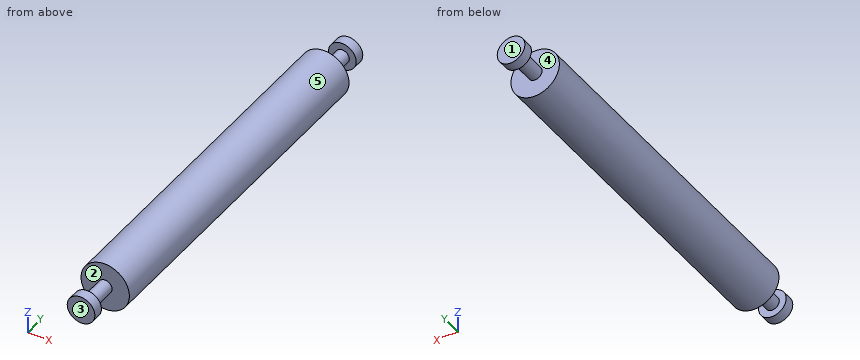
```python
from build123d import *

# Parameters (mm, degrees)
F0_R     = 3.5
F0_R_2   = 2
F0_R_3   = 1
F1_DEPTH = 25
F2_R     = 1
F3_DEPTH = 4
F4_W     = 1.5
F4_H     = 2


with BuildPart() as f1:
    # F0 (on Front) → F1 (new body)
    with BuildSketch(Plane.XZ):
        Circle(F0_R)
        Circle(F0_R_2, mode=Mode.SUBTRACT)
        Circle(F0_R_2)
        Circle(F0_R_3, mode=Mode.SUBTRACT)
        Circle(F0_R_3)
    extrude(amount=-F1_DEPTH)

    # F2 (on Front) → F3 (join)
    with BuildSketch(Plane.XZ):
        Circle(F2_R)
    extrude(amount=F3_DEPTH)

    # F4 (on Right) → F5 (revolve)
    with BuildSketch(Plane.YZ):
        with Locations((-4.75, 1)):
            Rectangle(F4_W, F4_H)
    revolve(axis=Axis((0, -4.75, 0), (0, 1, 0)))

    # F6: F1 across face


with BuildPart() as f1_1:
    add(f1.part)
    add(f1.part.mirror(Plane(origin=(0, 25, 0), x_dir=(1, 0, 0), z_dir=(0, 1, 0))))


solid = f1_1.part
```
Geometry: final body of the model. Coordinates: model frame, mm. Face numbers are marked on the shaded views. A direction names the side the tool comes from. Give positions to 0.01 mm unless a question says otherwise; leave off trailing zeros. Loops run counter-clockwise (first coordinate to the right, second up) from the corner with the lowest first, then second, coordinate; pieces in that order, holes last. Notation, with made-up numbers: (48, 84) - (91, 84) arc R14 ccw to (91, 101) - close; hole circle Ø4 at (59, -14.75). An arc over 180 degrees is marked (long way). Answer as CSV lines item,"result". Start each with the question number.
(1) Reachability of the marked faces 4 and 5 from +Z, -Z, +X, -X, +Y, -Y: full face, straight path, thin tool, end or side. Return the list, or none.
(2) Section query C-C (y = 35.5). Output: boundary loops of the cut face in (x, z).
(3) Pin query (flat end, axial travel): P1, Ø2, axis at y = 32.5, z = -2, coming from the -X side; P2, Ø1, axis at x = -2, z = -2.5, coming from the +Y side; P3, Ø2, axis at y = 11.5, z = 1.5, coming from the +X side. Return the tip coordinate at first contact, or that it passes through.
(4) Mould query, pull axis Y, two halves, no side actions, for the marked faces 1, 2 and 3. Classes: +Y half, -Y half, draft (parallel to the pull), parting line (faces both ways), or undercut.
(5) Section query A-A (x = 0). Output: boundary loops of the cut face in (y, z), and give its area (3 significant figures).
(6) Ray query, line 1 along Y through (x, z) = (-1.25, -0.75); line 2 along Y through (x, z) = (-2.5, -0.5); line 3 along Z through (x, y) = (0.25, 43). Return the intervals inside material, ascending. Write a range as [from, to].
(7) Section query B-B (z = -1.5). Output: boundary loops of the cut face in (x, y), and give its area (3 significant figures).
Worked answers:
1,face 4,"none"
1,face 5,"+Y, -Y"
2,outline,"circle Ø7 at (0, 0)"
3,P1,"stops at x = -3.35"
3,P2,"stops at y = 50"
3,P3,"stops at x = 3.46"
4,face 1,"+Y half"
4,face 2,"undercut"
4,face 3,"-Y half"
5,outline,"(-5.5, -2) - (-4, -2) - (-4, -1) - (0, -1) - (0, -3.5) - (50, -3.5) - (50, -1) - (54, -1) - (54, -2) - (55.5, -2) - (55.5, 2) - (54, 2) - (54, 1) - (50, 1) - (50, 3.5) - (0, 3.5) - (0, 1) - (-4, 1) - (-4, 2) - (-5.5, 2) - close"
5,area,"378 mm^2"
6,line 1,"y = [-5.5, -4], [0, 50], [54, 55.5]"
6,line 2,"y = [0, 50]"
6,line 3,"z = [-3.49, 3.49]"
7,outline,"(-3.16, 0) - (3.16, 0) - (3.16, 50) - (-3.16, 50) - close; (-1.32, -5.5) - (1.32, -5.5) - (1.32, -4) - (-1.32, -4) - close; (-1.32, 54) - (1.32, 54) - (1.32, 55.5) - (-1.32, 55.5) - close"
7,area,"324 mm^2"
